Geometry check sheet. Reference: drawing and pictorial views, mm from the part's lowest x, y, z. Give positions to 0.01 mm unless a question says otherwise; leave off trailing zeros. Write each loop counter-clockwise with the first axis right and the second up, starting at its lowest first coordinate (ties: lowest second). Pieces come first, ordered by that corner, then holes. Notation, with made-up numbers: (-36, -40) -> (-10, -40) arc R21 cw to (-10, -2) -> close; hole circle Ø9 at (-1.75, 5.5). An arc over 180 degrees is marked (long way). Use a Markdown table: item, result. Add a question column.
1. Cross-section at C-C (y = 1.8). Count the separate pieces of the cut face and the enclosed holes in it, then the cut area to 3 significant figures.
2. Scan lines: probe 1 along Z at (x, y) = (48, 2.55); probe 2 along X at (y, z) = (1.8, 6); probe 3 along Z at (x, y) = (28, 1.25). Record each from-to range of solid material in increasing order. Write a range as [from, to].
3. Cross-section at B-B (z = 6.6). Enter the section's corners in (x, y), then the cut area to 3 significant figures.
4. Cross-section at A-A (x = 53). Enter the section's corners in (y, z), then the cut area to 4 significant figures.
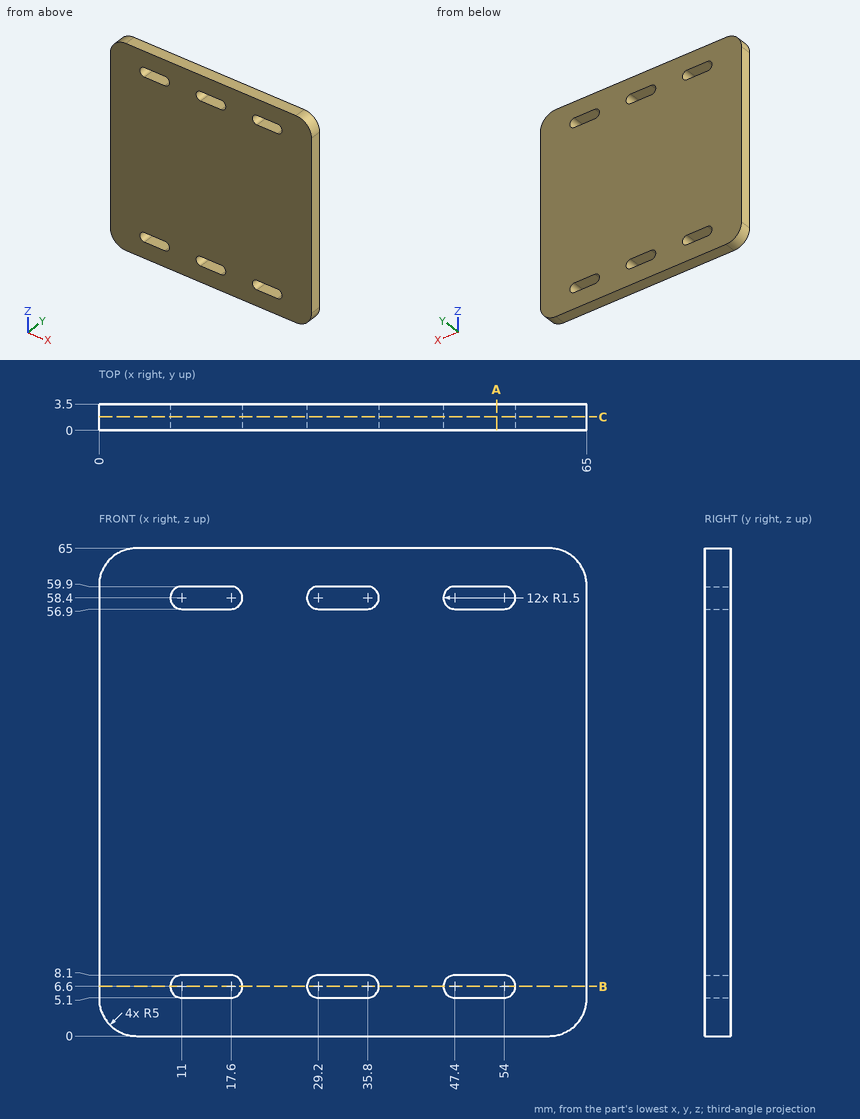
Worked answers:
| question | item | result |
|---|---|---|
| 1 | separate pieces | 1 |
| 1 | enclosed holes | 6 |
| 1 | area | 4,040 mm² |
| 2 | probe 1 | z = [0, 5.1], [8.1, 56.9], [59.9, 65] |
| 2 | probe 2 | x = [0, 9.63], [18.97, 27.83], [37.17, 46.03], [55.37, 65] |
| 2 | probe 3 | z = [0, 5.7], [7.5, 57.5], [59.3, 65] |
| 3 | outline | (0, 0) -> (9.5, 0) -> (9.5, 3.5) -> (0, 3.5) -> close; (19.1, 0) -> (27.7, 0) -> (27.7, 3.5) -> (19.1, 3.5) -> close; (37.3, 0) -> (45.9, 0) -> (45.9, 3.5) -> (37.3, 3.5) -> close; (55.5, 0) -> (65, 0) -> (65, 3.5) -> (55.5, 3.5) -> close |
| 3 | area | 127 mm² |
| 4 | outline | (0, 0) -> (3.5, 0) -> (3.5, 5.1) -> (0, 5.1) -> close; (0, 8.1) -> (3.5, 8.1) -> (3.5, 56.9) -> (0, 56.9) -> close; (0, 59.9) -> (3.5, 59.9) -> (3.5, 65) -> (0, 65) -> close |
| 4 | area | 206.5 mm² |
